Could you check a few things on this model? Use its own coordinates, in mm. A direction names the side the tool comes from. Coordinates: 2 decimals unless noted, no trailing zeros. Loops run counter-clockwise (first coordinate to the right, second up) from the corner with the lowest first, then second, coordinate; pieces in that order, holes last. Notation, with made-up numbers: (-11.75, 63.25) - (-4.75, 63.25) arc R26 cw to (-4.75, 92.25) - close; hole circle Ø7 at (-5, 51). An arc over 180 degrees is marked (long way). One line per item, written item: value. Start each with the question number.
(1) If I drill on line 1 along Z through (x, y) = (41, -26.5); line 2 along Z through (x, y) = (6, -11.5); line 3 along X through (y, z) = (-12, -16), over which ranges is the centre line in solid material (lowest first)? Write a range as from..to.
(2) If we section it at C-C on z = -22.5: Write out the boundary of the cut face in (x, y), then the cut area to 3 significant figures.
(3) I'm going to push flat-ended pins straight in: P1, Ø24, axis at x = 27.5, y = -36, coming from the -Z side; P2, Ø25, axis at x = 25, y = -30.5, coming from the +Z side; P3, Ø12, axis at y = -10, z = -22.5, coming from the +X side. Where does each tip first touch, or does it pass through?
(4) If we section it at A-A on y = -24: Write out the boundary of the cut face in (x, z).
(5) On a 3-axis mill with a long thin cutter (end or side, diameter ignored), from which of +Z, -Z, +X, -X, +Y, -Y can I reach the whole of each face in a straight line? I mean faces 1 (the face through (45, -25, -5)), 2 (the face through (20, -25, 0)), 3 (the face through (15, -25, -20)). Say none if no direction works.
(6) If we section it at B-B on x = -4: Write out the boundary of the cut face in (y, z).
```python
from build123d import *

# Parameters (mm, degrees)
F0_W     = 90
F0_H     = 60
F1_DEPTH = 50
F2_W     = 30
F2_H     = 50
F3_DEPTH = 20
F5_DEPTH = 50.001
F6_DEPTH = 50.001


with BuildPart() as f1:
    # F0 (on Front) → F1 (new body)
    with BuildSketch(Plane.XZ):
        Rectangle(F0_W, F0_H)
    extrude(amount=F1_DEPTH)

    # F2 (on face) → F3 (cut)
    with BuildSketch(Plane(origin=(0, 0, -30), x_dir=(1, 0, 0), z_dir=(0, 0, -1))):
        with Locations((30, 25)):
            Rectangle(F2_W, F2_H)
    extrude(amount=-F3_DEPTH, mode=Mode.SUBTRACT)

    # F4 (on face) → F5 (cut, through all)
    with BuildSketch(Plane(origin=(0, 0, 0), x_dir=(-1, 0, 0), z_dir=(0, 1, 0))):
        Polygon((45, 30), (25, 30), (45, 0), align=None)
    extrude(amount=-F5_DEPTH, mode=Mode.SUBTRACT)

    # F4 (on face) → F6 (cut, through all)
    with BuildSketch(Plane(origin=(0, 0, 0), x_dir=(-1, 0, 0), z_dir=(0, 1, 0))):
        Polygon((-45, 30), (-45, 0), (5, 0), (25, 30), align=None)
    extrude(amount=-F6_DEPTH, mode=Mode.SUBTRACT)


solid = f1.part
```
Values:
1. line 1: z = -10..0
1. line 2: z = -30..0
1. line 3: x = -45..15
2. outline: (-45, -50) - (15, -50) - (15, 0) - (-45, 0) - close
2. area: 3,000 mm2
3. P1: stops at z = -10
3. P2: stops at z = 0
3. P3: stops at x = 15
4. outline: (-45, -30) - (15, -30) - (15, -10) - (45, -10) - (45, 0) - (-5, 0) - (-25, 30) - (-45, 0) - close
5. face 1: +Z, -Z, +X, +Y, -Y
5. face 2: +Z, +X, +Y, -Y
5. face 3: -Z, +X, +Y, -Y
6. outline: (-50, -30) - (0, -30) - (0, 0) - (-50, 0) - close
